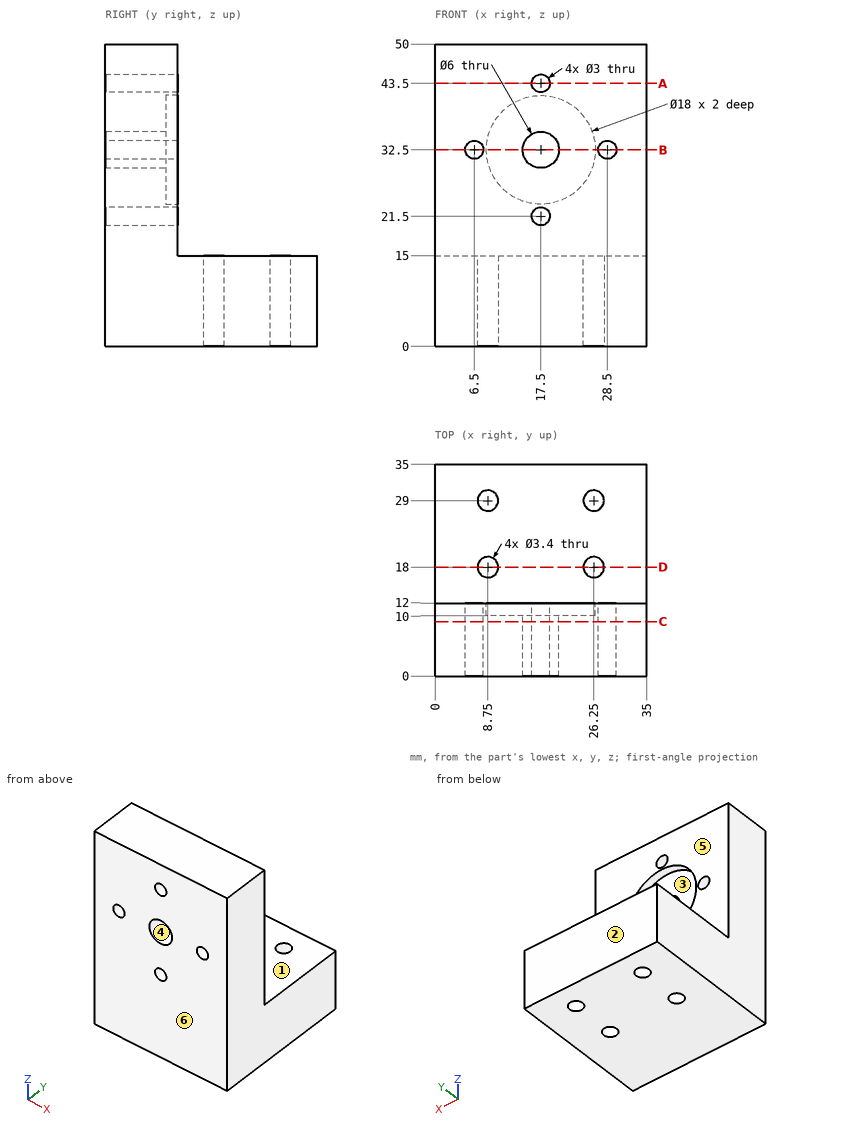
For this review, use the dimensioned drawing (mm, ordinates from the lowest corner) and the shaded views. A direction names the side the tool comes from. Give positions to 0.01 mm unless a question says otherwise; leave off trailing zeros. Write each loop counter-clockwise with the first axis right and the second up, starting at its lowest first coordinate (ties: lowest second). Pieces come first, ordered by that corner, then holes. Notation, with made-up numbers: M 13,-17 L 35,-17 A17 ccw 35,11 Z; hole C 4.25,86 d9. An arc over 180 degrees is marked long. Answer as a JSON object with one key per item and string values. Group by question number.
Item 1: Consider section D-D on y = 18. Write out the cut boundary in (x, z), plus the area to 3 significant figures.
Item 2: Consider section C-C on y = 9. Write out the cut boundary in (x, z), plus the area to 3 significant figures.
Item 3: Consider section B-B on z = 32.5. Write out the cut boundary in (x, y), plus the area to 3 significant figures.
Item 4: Draft analysis for pull direction Z (two halves, no side actions). For the marked faces 1, 2, 3 and 4, state which applies: +Z half, -Z half, draft (parallel to the pull), parting line (faces both ways), or undercut.
Item 5: Tool access review of the marked faces 5 and 6: name each direction out of +Z, -Z, +X, -X, +Y, -Y from which nothing blocks a thin tool from reaching the whole face with its end or side.
Item 6: For pin 1 Ø5.5 at (x, z) = (19, 34.5) entering from +Y; pin 2 Ø11.5 at (x, y) = (16, 23) entering from +Z, all flat-tipped, find the tip position at first contact; note any pin that passes through.
Item 7: For probe 1 along X at (y, z) = (3.25, 32.5); probe 2 along Y at (x, z) = (8.75, 8.5); probe 3 along Y at (x, z) = (25, 8.5), list the stretches that pass through material, from the lowest coordinate up. Write a range as [from, to].
Item 8: Consider section A-A on z = 43.5. Write out the cut boundary in (x, y).
Check result:
{
 "1": {"outline": "M 0,0 L 7.05,0 L 7.05,15 L 0,15 Z; M 10.45,0 L 24.55,0 L 24.55,15 L 10.45,15 Z; M 27.95,0 L 35,0 L 35,15 L 27.95,15 Z", "area": "423 mm^2"},
 "2": {"outline": "M 0,0 L 35,0 L 35,50 L 0,50 Z; hole C 6.5,32.5 d3; hole C 17.5,32.5 d6; hole C 17.5,21.5 d3; hole C 17.5,43.5 d3; hole C 28.5,32.5 d3", "area": "1,690 mm^2"},
 "3": {"outline": "M 0,0 L 5,0 L 5,12 L 0,12 Z; M 8,0 L 14.5,0 L 14.5,10 L 8.5,10 L 8.5,12 L 8,12 Z; M 20.5,0 L 27,0 L 27,12 L 26.5,12 L 26.5,10 L 20.5,10 Z; M 30,0 L 35,0 L 35,12 L 30,12 Z", "area": "252 mm^2"},
 "4": {"face 1": "+Z half", "face 2": "draft", "face 3": "undercut", "face 4": "undercut"},
 "5": {"face 5": "+Z, +X, -X, +Y", "face 6": "+Z, -Z, +X, -X, -Y"},
 "6": {"pin 1": "stops at y = 10", "pin 2": "stops at z = 15"},
 "7": {"probe 1": "x = [0, 5], [8, 14.5], [20.5, 27], [30, 35]", "probe 2": "y = [0, 16.3], [19.7, 27.3], [30.7, 35]", "probe 3": "y = [0, 16.85], [19.15, 27.85], [30.15, 35]"},
 "8": {"outline": "M 0,0 L 16,0 L 16,12 L 0,12 Z; M 19,0 L 35,0 L 35,12 L 19,12 Z"}
}
